from build123d import *

# Parameters (mm, degrees)
SKETCH1_R           = 2
SKETCH1_R_2         = 3
BOSS_EXTRUDE1_DEPTH = 2
SKETCH3_R           = 10
SKETCH3_R_2         = 2
CUT_EXTRUDE1_DEPTH  = 93.316865626
CUT_EXTRUDE2_DEPTH  = 93.316865626
CUT_EXTRUDE3_DEPTH  = 93.316865626
FILLET1_R           = 2
FILLET2_DEPTH       = 2
FILLET3_DEPTH       = 2
FILLET4_DEPTH       = 2
FILLET5_DEPTH       = 2
FILLET6_R           = 10
CUT_EXTRUDE4_START  = -10
CUT_EXTRUDE4_DEPTH  = 10
FILLET7_R           = 4


with BuildPart() as part:
    # Sketch1 → Boss-Extrude1 (new body)
    with BuildSketch(Plane.XY):
        with BuildLine():
            Line((-73.916912814, -12.7), (-15.450242717, -12.7))
            ThreePointArc((-15.450242717, -12.7), (0, -20), (15.450242717, -12.7))
            Line((15.450242717, -12.7), (73.916912814, -12.7))
            ThreePointArc((73.916912814, -12.7), (75, 0), (73.916912814, 12.7))
            Line((73.916912814, 12.7), (53.192030909, 51.162152625))
            ThreePointArc((53.192030909, 51.162152625), (51.353674008, 53.083322806), (48.790367902, 53.790367902))
            Line((48.790367902, 53.790367902), (-48.790367902, 53.790367902))
            ThreePointArc((-48.790367902, 53.790367902), (-51.353674008, 53.083322806), (-53.192030909, 51.162152625))
            Line((-53.192030909, 51.162152625), (-73.916912814, 12.7))
            ThreePointArc((-73.916912814, 12.7), (-75, 0), (-73.916912814, -12.7))
        make_face()
        with Locations((0, 15)):
            Circle(SKETCH1_R, mode=Mode.SUBTRACT)
        with Locations((15, 0)):
            Circle(SKETCH1_R, mode=Mode.SUBTRACT)
        with Locations((0, -15)):
            Circle(SKETCH1_R, mode=Mode.SUBTRACT)
        with Locations((-15, 0)):
            Circle(SKETCH1_R, mode=Mode.SUBTRACT)
        with Locations((-48.790367902, 48.790367902)):
            Circle(SKETCH1_R_2, mode=Mode.SUBTRACT)
        with Locations((-69, 0)):
            Circle(SKETCH1_R_2, mode=Mode.SUBTRACT)
        with Locations(Location((69, 0, 0), (0, 0, 180))):
            Circle(SKETCH1_R_2, mode=Mode.SUBTRACT)
        with Locations(Location((48.790367902, 48.790367902, 0), (0, 0, 180))):
            Circle(SKETCH1_R_2, mode=Mode.SUBTRACT)
    extrude(amount=BOSS_EXTRUDE1_DEPTH)

    # Sketch3 → Cut-Extrude1 (cut, through all)
    with BuildSketch(Plane(origin=(0, 0, 0), x_dir=(-1, 0, 0), z_dir=(0, 0, -1))):
        Circle(SKETCH3_R)
        with Locations((-57, 0)):
            Circle(SKETCH3_R_2)
        with Locations((-32, 0)):
            Circle(SKETCH3_R_2)
        with Locations((-23.5, 0)):
            Circle(SKETCH3_R_2)
        with Locations(Location((23.5, 0, 0), (0, 0, 180))):
            Circle(SKETCH3_R_2)
        with Locations(Location((32, 0, 0), (0, 0, 180))):
            Circle(SKETCH3_R_2)
        with Locations(Location((57, 0, 0), (0, 0, 180))):
            Circle(SKETCH3_R_2)
    extrude(amount=-CUT_EXTRUDE1_DEPTH, mode=Mode.SUBTRACT)

    # Sketch5 → Cut-Extrude2 (cut, through all)
    with BuildSketch(Plane.XY.offset(2)):
        with BuildLine():
            ThreePointArc((-47.496272676, 43.96073877), (-49.370145809, 43.824095902), (-51.162152637, 44.388704901))
            Line((-51.162152637, 44.388704901), (-66.890145502, 15.2))
            Line((-66.890145502, 15.2), (-18.735533906, 15.2))
            Line((-18.735533906, 15.2), (-47.496272676, 43.96073877))
        make_face()
        with BuildLine():
            ThreePointArc((43.96073877, 47.496272676), (43.833143595, 48.137736941), (43.790367902, 48.790367902))
            Line((43.790367902, 48.790367902), (-43.790367902, 48.790367902))
            ThreePointArc((-43.790367902, 48.790367902), (-43.833143595, 48.137736941), (-43.96073877, 47.496272676))
            Line((-43.96073877, 47.496272676), (-12.263448247, 15.798982153))
            ThreePointArc((-12.263448247, 15.798982153), (0, 20), (12.263448247, 15.798982153))
            Line((12.263448247, 15.798982153), (43.96073877, 47.496272676))
        make_face()
        with BuildLine():
            Line((47.496272676, 43.96073877), (18.735533906, 15.2))
            Line((18.735533906, 15.2), (66.886464241, 15.2))
            Line((66.886464241, 15.2), (51.159299215, 44.387168561))
            ThreePointArc((51.159299215, 44.387168561), (49.368536342, 43.823908272), (47.496272676, 43.96073877))
        make_face()
    extrude(amount=-CUT_EXTRUDE2_DEPTH, mode=Mode.SUBTRACT)

    # Sketch8 → Cut-Extrude3 (cut, through all)
    with BuildSketch(Plane.XY.offset(2)):
        with BuildLine():
            Line((61.58620553, 10.2), (20, 10.2))
            ThreePointArc((20, 10.2), (17.4, 7.6), (20, 5))
            Line((20, 5), (61.58620553, 5))
            ThreePointArc((61.58620553, 5), (64.18620553, 7.6), (61.58620553, 10.2))
        make_face()
        with BuildLine():
            Line((-61.58620553, -10.2), (-20, -10.2))
            ThreePointArc((-20, -10.2), (-17.4, -7.6), (-20, -5))
            Line((-20, -5), (-61.58620553, -5))
            ThreePointArc((-61.58620553, -5), (-64.18620553, -7.6), (-61.58620553, -10.2))
        make_face()
        with BuildLine():
            Line((61.58620553, -10.2), (20, -10.2))
            ThreePointArc((20, -10.2), (17.4, -7.6), (20, -5))
            Line((20, -5), (61.58620553, -5))
            ThreePointArc((61.58620553, -5), (64.18620553, -7.6), (61.58620553, -10.2))
        make_face()
        with BuildLine():
            Line((-61.58620553, 10.2), (-20, 10.2))
            ThreePointArc((-20, 10.2), (-17.4, 7.6), (-20, 5))
            Line((-20, 5), (-61.58620553, 5))
            ThreePointArc((-61.58620553, 5), (-64.18620553, 7.6), (-61.58620553, 10.2))
        make_face()
    extrude(amount=-CUT_EXTRUDE3_DEPTH, mode=Mode.SUBTRACT)

    # Fillet1
    fillet1_edges = [part.edges().sort_by_distance(p)[0] for p in [
        (12.263448247, 15.798982153, 1),
        (-12.263448247, 15.798982153, 1),
        (66.886464241, 15.2, 1),
        (18.735533906, 15.2, 1),
        (-18.735533906, 15.2, 1),
        (-66.890145502, 15.2, 1),
        (-15.450242717, -12.7, 1),
        (15.450242717, -12.7, 1),
    ]]
    fillet(fillet1_edges, radius=FILLET1_R)

    # Fillet2: read off the stored shape, not the designer's step
    # Fillet2 outline → Fillet2 (add)
    with BuildSketch(Plane.XY):
        with BuildLine():
            Line((-43.96073877, 47.496272676), (-43.584387401, 47.119921307))
            add(Edge.make_bspline(
                [(-43.584387401, 47.119921307), (-43.79719002, 47.332723926), (-43.913795032, 47.634492314), (-43.857793188, 47.97201181)],
                knots=[0, 0, 0, 0, 0.414217666, 0.414217666, 0.414217666, 0.414217666], degree=3, weights=[1, 0.829531048, 0.729673348, 0.700426898]))
            ThreePointArc((-43.857793188, 47.97201181), (-43.903473396, 47.732888781), (-43.96073877, 47.496272676))
        make_face()
        with BuildLine():
            ThreePointArc((-43.790367902, 48.790367902), (-43.807252733, 48.379803393), (-43.857793188, 47.97201181))
            add(Edge.make_bspline(
                [(-43.857793188, 47.97201181), (-43.770111484, 48.500463775), (-43.357659279, 48.790367902), (-42.892465766, 48.790367902)],
                knots=[0.414217666, 0.414217666, 0.414217666, 0.414217666, 1, 1, 1, 1], degree=3, weights=[0.700426898, 0.659066873, 0.758924573, 1]))
            Line((-42.892465766, 48.790367902), (-43.790367902, 48.790367902))
        make_face()
    extrude(amount=FILLET2_DEPTH)

    # Fillet3: read off the stored shape, not the designer's step
    # Fillet3 outline → Fillet3 (add)
    with BuildSketch(Plane.XY):
        with BuildLine():
            Line((43.790367902, 48.790367902), (42.892465766, 48.790367902))
            add(Edge.make_bspline(
                [(42.892465766, 48.790367902), (43.357665683, 48.790367902), (43.770121408, 48.5004568), (43.857795774, 47.971996226)],
                knots=[0, 0, 0, 0, 0.585788454, 0.585788454, 0.585788454, 0.585788454], degree=3, weights=[1, 0.758922055, 0.659064787, 0.700428195]))
            ThreePointArc((43.857795774, 47.971996226), (43.807253382, 48.379795521), (43.790367902, 48.790367902))
        make_face()
        with BuildLine():
            ThreePointArc((43.96073877, 47.496272676), (43.903475067, 47.732881061), (43.857795774, 47.971996226))
            add(Edge.make_bspline(
                [(43.857795774, 47.971996226), (43.913791115, 47.634482177), (43.79718623, 47.332720136), (43.584387401, 47.119921307)],
                knots=[0.585788454, 0.585788454, 0.585788454, 0.585788454, 1, 1, 1, 1], degree=3, weights=[0.700428195, 0.729676298, 0.829533567, 1]))
            Line((43.584387401, 47.119921307), (43.96073877, 47.496272676))
        make_face()
    extrude(amount=FILLET3_DEPTH)

    # Fillet4: read off the stored shape, not the designer's step
    # Fillet4 outline → Fillet4 (add)
    with BuildSketch(Plane.XY):
        with BuildLine():
            Line((-51.162152637, 44.388704901), (-52.646203675, 41.634537337))
            add(Edge.make_bspline(
                [(-52.646203675, 41.634537337), (-51.92183636, 42.978850243), (-50.576640467, 43.835721987), (-48.922136441, 43.792104498)],
                knots=[0, 0, 0, 0, 0.585786442, 0.585786442, 0.585786442, 0.585786442], degree=3, weights=[1, 0.842637329, 0.777455577, 0.804454744]))
            ThreePointArc((-48.922136441, 43.792104498), (-50.077196468, 43.958797532), (-51.162152637, 44.388704901))
        make_face()
        with BuildLine():
            ThreePointArc((-47.496272676, 43.96073877), (-48.203119904, 43.824973679), (-48.922136441, 43.792104498))
            add(Edge.make_bspline(
                [(-48.922136441, 43.792104498), (-47.817700519, 43.762988388), (-46.849981733, 43.314447827), (-46.126053502, 42.590519596)],
                knots=[0.585786442, 0.585786442, 0.585786442, 0.585786442, 1, 1, 1, 1], degree=3, weights=[0.804454744, 0.823546038, 0.88872779, 1]))
            Line((-46.126053502, 42.590519596), (-47.496272676, 43.96073877))
        make_face()
    extrude(amount=FILLET4_DEPTH)

    # Fillet5: read off the stored shape, not the designer's step
    # Fillet5 outline → Fillet5 (add)
    with BuildSketch(Plane.XY):
        with BuildLine():
            Line((47.496272676, 43.96073877), (46.127063611, 42.591529705))
            add(Edge.make_bspline(
                [(46.127063611, 42.591529705), (46.850510453, 43.314976547), (47.817619792, 43.763154251), (48.921332432, 43.792083367)],
                knots=[0, 0, 0, 0, 0.414289791, 0.414289791, 0.414289791, 0.414289791], degree=3, weights=[1, 0.888707311, 0.823522047, 0.804444208]))
            ThreePointArc((48.921332432, 43.792083367), (48.202720546, 43.825020926), (47.496272676, 43.96073877))
        make_face()
        with BuildLine():
            ThreePointArc((51.159299215, 44.387168561), (50.075241983, 43.958277402), (48.921332432, 43.792083367))
            add(Edge.make_bspline(
                [(48.921332432, 43.792083367), (50.574149341, 43.835404908), (51.917905025, 42.979314342), (52.641529007, 41.636380946)],
                knots=[0.414289791, 0.414289791, 0.414289791, 0.414289791, 1, 1, 1, 1], degree=3, weights=[0.804444208, 0.777472544, 0.842657808, 1]))
            Line((52.641529007, 41.636380946), (51.159299215, 44.387168561))
        make_face()
    extrude(amount=FILLET5_DEPTH)

    # Fillet6
    fillet6_edges = [part.edges().sort_by_distance(p)[0] for p in [
        (-73.916912814, -12.7, 1),
        (73.916912814, -12.7, 1),
    ]]
    fillet(fillet6_edges, radius=FILLET6_R)

    # Sketch9 → Cut-Extrude4 (cut)
    with BuildSketch(Plane.XY.offset(2).offset(CUT_EXTRUDE4_START)):
        with BuildLine():
            Line((72.569817001, 15.2), (53.192030909, 51.162152625))
            ThreePointArc((53.192030909, 51.162152625), (51.353674008, 53.083322806), (48.790367902, 53.790367902))
            Line((48.790367902, 53.790367902), (-48.790367902, 53.790367902))
            ThreePointArc((-48.790367902, 53.790367902), (-51.353674008, 53.083322806), (-53.192030909, 51.162152625))
            Line((-53.192030909, 51.162152625), (-72.569817001, 15.2))
            Line((-72.569817001, 15.2), (-12.998461447, 15.2))
            ThreePointArc((-12.998461447, 15.2), (0, 20), (12.998461447, 15.2))
            Line((12.998461447, 15.2), (72.569817001, 15.2))
        make_face()
    extrude(amount=CUT_EXTRUDE4_DEPTH, mode=Mode.SUBTRACT)

    # Fillet7
    fillet7_edges = [part.edges().sort_by_distance(p)[0] for p in [
        (-72.569817001, 15.2, 1),
        (72.569817001, 15.2, 1),
        (-12.998461447, 15.2, 1),
        (12.998461447, 15.2, 1),
    ]]
    fillet(fillet7_edges, radius=FILLET7_R)


solid = part.part
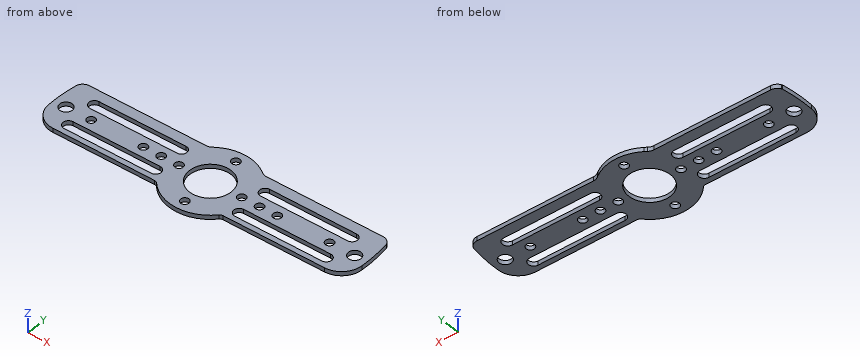
CAD build for the part. Positions are in the model's coordinates, mm. Round coordinates to 2 decimals unless told otherwise and drop trailing zeros. Order: outer loops, then holes, each group sorted by start corner. A loop starts at its lowest first (then second) coordinate and runs counter-clockwise, first axis right, second up. Notation, with made-up numbers: (60, 28.5) -> (78, 28.5) arc R14 cw to (78, 36.5) -> close; hole circle Ø6 at (47, 3). An arc over 180 degrees is marked (long way). Write each question's results on one line, items separated by ' | '.
1. Flat gauge pins, fed straight in: P1, Ø0.6, axis at x = -41, z = 1, coming from the +Y side; P2, Ø5, axis at x = 23.5, y = 0, coming from the +Z side; P3, Ø2.5, axis at x = 0, y = -15, coming from the +Z side; P4, Ø1, axis at x = -29, z = 0.5, coming from the -Y side. Where does each tip first touch, or does it go through?
Findings below:
P1: stops at y = 15.2 | P2: stops at z = 2 | P3: passes through | P4: stops at y = -12.7
2. Cut at C-C (z = 0.8). Count the separate pieces of the cut face and the enclosed holes in it, plus the area to 3 significant figures.
Findings below:
separate pieces: 1 | enclosed holes: 17 | area: 2,920 mm²
3. Cut at A-A (x = 23.5). Give the cut face in (y, z), plus the area to 3 significant figures.
Findings below:
outline: (-12.7, 0) -> (-10.2, 0) -> (-10.2, 2) -> (-12.7, 2) -> close; (-5, 0) -> (-2, 0) -> (-2, 2) -> (-5, 2) -> close; (2, 0) -> (5, 0) -> (5, 2) -> (2, 2) -> close; (10.2, 0) -> (15.2, 0) -> (15.2, 2) -> (10.2, 2) -> close | area: 27.0 mm²
4. Cut at B-B (y = -7.6). Give the cut face in (x, z), plus the area to 3 significant figures.
Findings below:
outline: (-73.66, 0) -> (-64.19, 0) -> (-64.19, 2) -> (-73.66, 2) -> close; (-17.4, 0) -> (-6.5, 0) -> (-6.5, 2) -> (-17.4, 2) -> close; (6.5, 0) -> (17.4, 0) -> (17.4, 2) -> (6.5, 2) -> close; (64.19, 0) -> (73.66, 0) -> (73.66, 2) -> (64.19, 2) -> close | area: 81.5 mm²
5. Wall check: line 1 along Y through (x, z) = (-23.5, 1.25); line 2 along Y through (x, z) = (-41.5, 1.2); line 3 along X through (y, z) = (-8.5, 1.9). Give the ranges that are in metal, low to high. Write a range as [from, to].
Findings below:
line 1: y = [-12.7, -10.2], [-5, -2], [2, 5], [10.2, 15.2] | line 2: y = [-12.7, -10.2], [-5, 5], [10.2, 15.2] | line 3: x = [-73.09, -64.03], [-17.56, -5.27], [5.27, 17.56], [64.03, 73.09]
